Input: dimensioned drawing with shaded views. Units: mm. Origin: part minimum x, y, z. A direction names the side the tool comes from. Give positions to 0.01 mm unless a question says otherwise; leave off trailing zeros. Write each loop counter-clockwise with the first axis right and the second up, starting at its lowest first coordinate (ties: lowest second). Pieces come first, ordered by that corner, then holes. Notation, with made-up numbers: (48.25, 45) -> (58.25, 45) arc R33 cw to (58.25, 77) -> close; hole circle Ø3 at (77, -15.5). An arc over 180 degrees is marked (long way). Answer in a Markdown table with one row per item. Add a question column.
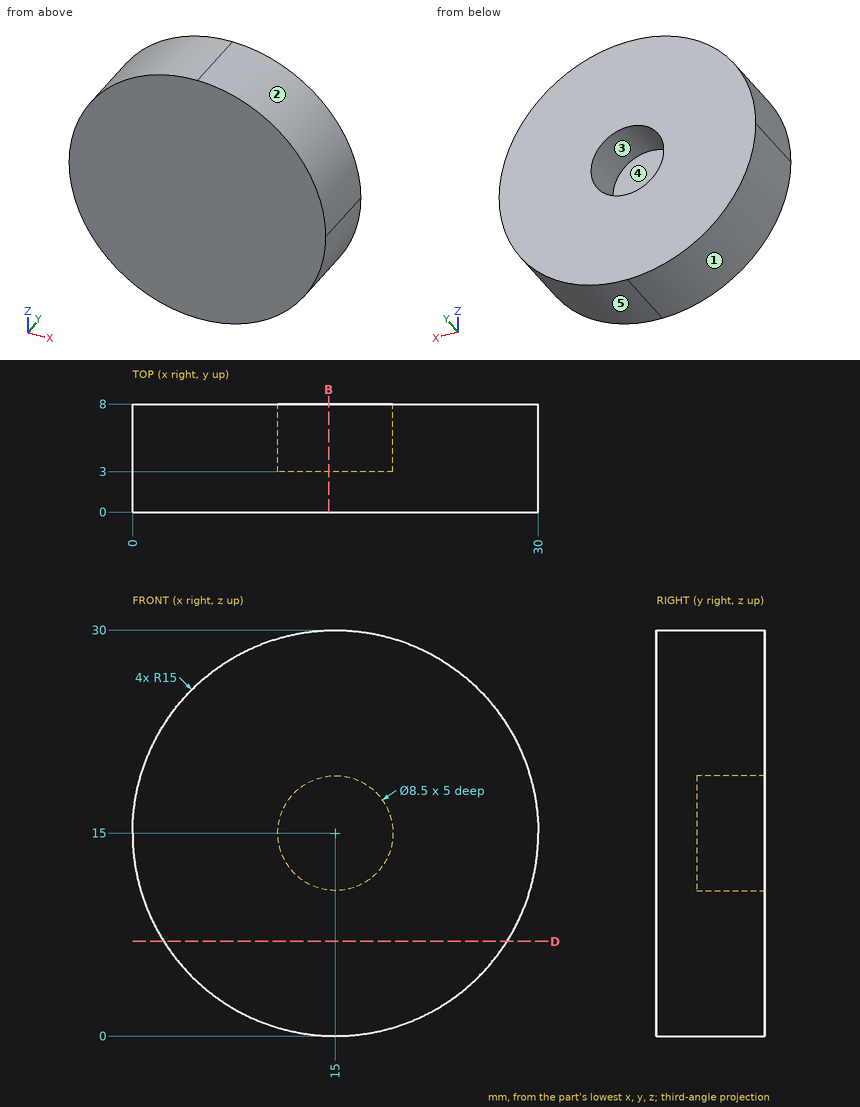
Q1. Access query for the marked faces 4 and 5. Directions: +Z, -Z, +X, -X, +Y, -Y. A direction counts if a zero-diameter tool reaches every point of the face in a straight line with its end or side. Return the directions, or none.
Q2. Pull-direction query (X, two-part tool) for the marked faces 1, 2 and 3; classes: +X half, -X half, draft (parallel to the pull), parting line (faces both ways), or undercut.
Q3. Line query: probe 1 along X at (y, z) = (4.95, 15); probe 2 along Y at (x, z) = (17.5, 13); probe 3 along X at (y, z) = (2, 5). Output: solid intervals per line, ascending. Write a range as from..to.
Q4. Section D-D on z = 7. Return loops of the section in (x, y).
Q5. Section B-B on x = 14.5. Return loops of the section in (y, z).
Q6. Contact query for flat-ended pins moving along their axis: pin 1 Ø2 at (x, y) = (25.5, 2) entering from -Z; pin 2 Ø1.5 at (x, z) = (24.5, 10) entering from -Y; pin 3 Ø1.5 at (x, y) = (22, 3.5) entering from -Z; pin 4 Ø1.5 at (y, z) = (4, 5.5) entering from +X. Output: stop coordinate, or through.
Checks:
| question | item | result |
|---|---|---|
| 1 | face 4 | +Y |
| 1 | face 5 | -Z, +X, +Y, -Y |
| 2 | face 1 | -X half |
| 2 | face 2 | +X half |
| 2 | face 3 | undercut |
| 3 | probe 1 | 0..10.75, 19.25..30 |
| 3 | probe 2 | 0..3 |
| 3 | probe 3 | 3.82..26.18 |
| 4 | outline | (2.31, 0) -> (27.69, 0) -> (27.69, 8) -> (2.31, 8) -> close |
| 5 | outline | (0, 0.01) -> (8, 0.01) -> (8, 10.78) -> (3, 10.78) -> (3, 19.22) -> (8, 19.22) -> (8, 29.99) -> (0, 29.99) -> close |
| 6 | pin 1 | z = 3.39 |
| 6 | pin 2 | y = 0 |
| 6 | pin 3 | z = 1.36 |
| 6 | pin 4 | x = 27.18 |
